Verification items for the finished model (mm, model axes). Face numbers are marked on the shaded views. A direction names the side the tool comes from. Coordinates: 2 decimals unless noted, no trailing zeros. Order: outer loops, then holes, each group sorted by start corner. A loop starts at its lowest first (then second) coordinate and runs counter-clockwise, first axis right, second up. Notation, with made-up numbers: (83, 38) - (124, 38) arc R21 cw to (124, 60) - close; hole circle Ø4 at (80, 82). An arc over 180 degrees is marked (long way). Answer as CSV lines item,"result". Start each with the question number.
1. Section check A-A (y = 180). Record the cut outline in (x, z).
2. Section check C-C (x = 203). Record the cut outline in (y, z).
3. Material ranges on L1, parallel to X at y = -223.65, z = -450; L2, parallel to Z at x = -169.55, y = -222.75; L3, parallel to Y at x = -3, z = -513, recorded low to high. Write a range as [from, to].
4. Section check B-B (z = -361.5). Record the cut outline in (x, y), and give its area (3 significant figures).
5. Go/stop test with flat-tipped pins: pin 1 (6.5 mm diameter, centred on x = -169.55, z = -424, fed in from -Y); pin 2 (1 mm diameter, centred on x = -87.5, z = -193.5, fed in from -Y). Record where each tip stops, or that it passes through.
6. Section check D-D (x = -127). Record the cut outline in (y, z).
7. Mould release check, pull along X, two halves, no side actions. Record for the marked faces 3, 4 and 5: pulls with the +X half, pulls with the -X half, needs draft (parallel to the pull), parting line crosses it, or undercut.
8. Set-up check for the marked faces 1 and 2: record each of +Z, -Z, +X, -X, +Y, -Y from which the full face is reachable in a straight line by a thin tool's end or side.
from build123d import *

# Parameters (mm, degrees)
SKETCH1_W           = 520
SKETCH1_H           = 450
BOSS_EXTRUDE1_DEPTH = 5
BOSS_EXTRUDE3_DEPTH = 560
SKETCH4_W           = 520
SKETCH4_H           = 450
BOSS_EXTRUDE4_DEPTH = 5
SKETCH5_W           = 520
SKETCH5_H           = 450
SKETCH5_W_2         = 510
SKETCH5_H_2         = 440
BOSS_EXTRUDE5_DEPTH = 100
SKETCH6_R           = 2.5
CUT_EXTRUDE1_DEPTH  = 10


with BuildPart() as part:
    # Sketch1 → Boss-Extrude1 (new body)
    with BuildSketch(Plane.XY):
        Rectangle(SKETCH1_W, SKETCH1_H)
    extrude(amount=BOSS_EXTRUDE1_DEPTH)

    # Sketch3 → Boss-Extrude3 (add)
    with BuildSketch(Plane(origin=(0, 0, 0), x_dir=(-1, 0, 0), z_dir=(0, 0, -1))):
        Polygon((260, 225), (-260, 225), (-260, -225), (-155, -225), (-155, -220), (-255, -220), (-255, 220), (255, 220), (255, -220), (155, -220), (155, -225), (260, -225), align=None)
    extrude(amount=BOSS_EXTRUDE3_DEPTH)

    # Sketch4 → Boss-Extrude4 (add)
    with BuildSketch(Plane(origin=(0, 0, -560), x_dir=(-1, 0, 0), z_dir=(0, 0, -1))):
        Rectangle(SKETCH4_W, SKETCH4_H)
    extrude(amount=BOSS_EXTRUDE4_DEPTH)

    # Sketch5 → Boss-Extrude5 (add)
    with BuildSketch(Plane.XY.offset(-560)):
        Rectangle(SKETCH5_W, SKETCH5_H)
        Rectangle(SKETCH5_W_2, SKETCH5_H_2, mode=Mode.SUBTRACT)
    extrude(amount=BOSS_EXTRUDE5_DEPTH)

    # Sketch6 → Cut-Extrude1 (cut)
    with BuildSketch(Plane.XZ.offset(225)):
        with Locations((-169.55, -10)):
            Circle(SKETCH6_R)
        with Locations((-169.55, -36)):
            Circle(SKETCH6_R)
        with Locations((-169.55, -450)):
            Circle(SKETCH6_R)
        with Locations((-169.55, -424)):
            Circle(SKETCH6_R)
    extrude(amount=-CUT_EXTRUDE1_DEPTH, mode=Mode.SUBTRACT)


solid = part.part
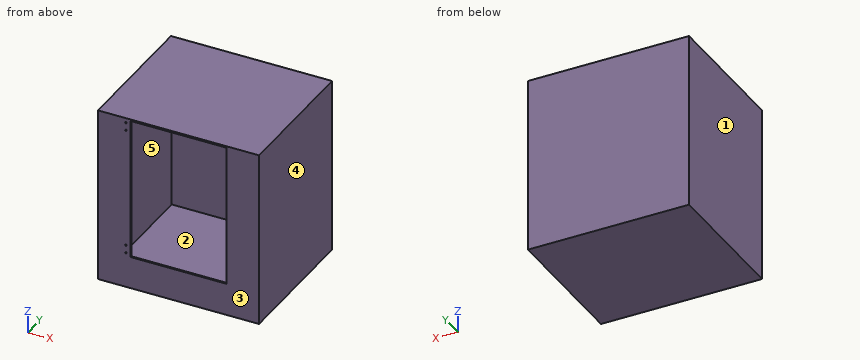
Evaluation:
1,outline,"(-260, -565) - (260, -565) - (260, 5) - (-260, 5) - close; hole (-255, -560) - (255, -560) - (255, 0) - (-255, 0) - close"
2,outline,"(-225, -565) - (225, -565) - (225, 5) - (-225, 5) - close; hole (-220, -560) - (220, -560) - (220, 0) - (-220, 0) - close"
3,L1,"x = [-260, -172.05], [-167.05, -155], [155, 260]"
3,L2,"z = [-565, -452.5], [-447.5, -426.5], [-421.5, -38.5], [-33.5, -12.5], [-7.5, 5]"
3,L3,"y = [-225, -220], [220, 225]"
4,outline,"(-260, -225) - (-155, -225) - (-155, -220) - (-255, -220) - (-255, 220) - (255, 220) - (255, -220) - (155, -220) - (155, -225) - (260, -225) - (260, 225) - (-260, 225) - close"
4,area,"8,050 mm²"
5,pin 1,"stops at y = -225"
5,pin 2,"stops at y = 220"
6,outline,"(-225, -565) - (225, -565) - (225, 5) - (-225, 5) - (-225, 0) - (220, 0) - (220, -560) - (-220, -560) - (-220, -460) - (-225, -460) - close"
7,face 3,"needs draft"
7,face 4,"pulls with the +X half"
7,face 5,"undercut"
8,face 1,"+Z, -Z, -X, +Y, -Y"
8,face 2,"none"
